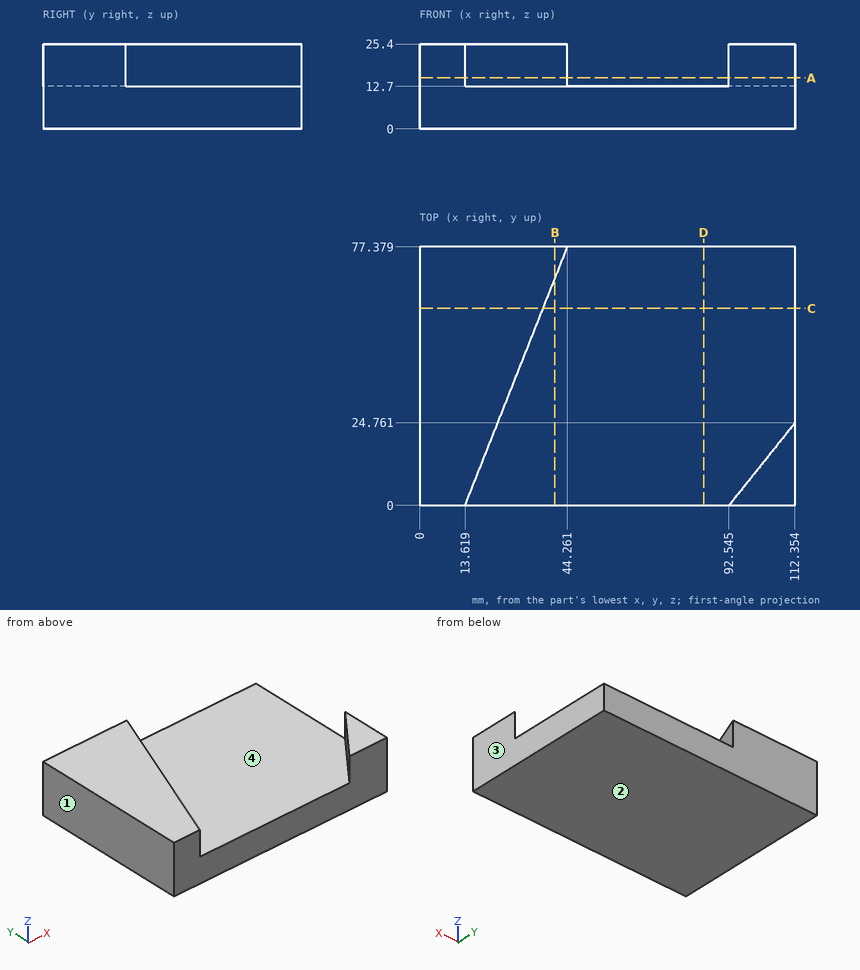
Print and shaded views of the part. All mm, measured from the part's lowest x, y and z. Round coordinates to 2 decimals unless told otherwise and drop trailing zeros. Write each loop counter-clockwise with the first axis right and the second up, starting at its lowest first coordinate (ties: lowest second). Pieces come first, ordered by that corner, then holes. Notation, with made-up numbers: (40, -32) -> (61, -32) arc R19 cw to (61, -27) -> close; hole circle Ø1 at (8.25, -19). An arc over 180 degrees is marked (long way). Answer in a Markdown table with one row per item. Add a question column.
Item 1: Drop flat-ended pins along their axis: pin 1 Ø4 at (y, z) = (66.5, 15) entering from -X; pin 2 Ø2 at (x, y) = (55.5, 32) entering from +Z. Give the stop position or say it passes through.
Item 2: Saw through at B-B, the plane x = 40.5. Write the cut outline in (y, z), then the cut area to 3 significant figures.
Item 3: Drill centre lines: line 1 (Z direction, x = 38.5, y = 34); line 2 (Y direction, x = 97, z = 15.5) (1 decimal); line 3 (X direction, y = 38.5, z = 19.5) (1 decimal). Where is each one in solid material? Low to high. Write a range as from..to.
Item 4: Mould opens along X. For the marked faces 1, 2, 3 and 4 say: pulls with the +X half, pulls with the -X half, needs draft (parallel to the pull), parting line crosses it, or undercut.
Item 5: Saw through at D-D, the plane x = 85. Write the cut outline in (y, z), then the cut area to 3 significant figures.
Item 6: Saw through at A-A, the plane z = 15.25. Write the cut outline in (x, y) (1 decimal).
Item 7: Saw through at C-C, the plane y = 59. Write the cut outline in (x, z) (1 decimal).
Findings below:
| question | item | result |
|---|---|---|
| 1 | pin 1 | stops at x = 0 |
| 1 | pin 2 | stops at z = 12.7 |
| 2 | outline | (0, 0) -> (77.38, 0) -> (77.38, 25.4) -> (67.88, 25.4) -> (67.88, 12.7) -> (0, 12.7) -> close |
| 2 | area | 1,100 mm^2 |
| 3 | line 1 | z = 0..12.7 |
| 3 | line 2 | y = 0..5.6 |
| 3 | line 3 | x = 0..28.9 |
| 4 | face 1 | pulls with the -X half |
| 4 | face 2 | needs draft |
| 4 | face 3 | pulls with the +X half |
| 4 | face 4 | undercut |
| 5 | outline | (0, 0) -> (77.38, 0) -> (77.38, 12.7) -> (0, 12.7) -> close |
| 5 | area | 983 mm^2 |
| 6 | outline | (0, 0) -> (13.6, 0) -> (44.3, 77.4) -> (0, 77.4) -> close; (92.5, 0) -> (112.4, 0) -> (112.4, 24.8) -> close |
| 7 | outline | (0, 0) -> (112.4, 0) -> (112.4, 12.7) -> (37, 12.7) -> (37, 25.4) -> (0, 25.4) -> close |
